Verification items for the finished model (mm, model axes). Coordinates: 2 decimals unless noted, no trailing zeros. Order: outer loops, then holes, each group sorted by start corner. A loop starts at its lowest first (then second) coordinate and runs counter-clockwise, first axis right, second up. Notation, with made-up numbers: (27.25, 48.5) - (68.25, 48.5) arc R11 ccw to (68.25, 69.5) - close; hole circle Ø7 at (2.25, -6.5). An arc over 180 degrees is marked (long way). Answer as CSV lines item,"result". Start each with the question number.
1. Material ranges on L1, parallel to Y at x = 42.5, z = 11.5; L2, parallel to Y at x = 49, z = 11; L3, parallel to X at y = 36, z = 4 (3 decimals), recorded low to high. Write a range as [from, to].
2. Section check B-B (y = 24). Record the cut outline in (x, z), and give its area (3 significant figures).
3. Section check C-C (x = 44). Record the cut outline in (y, z), and give its area (3 significant figures).
4. Go/stop test with flat-tipped pins: pin 1 (1.5 mm diameter, centred on x = 63, z = 41.5, fed in from +Y); pin 2 (10 mm diameter, centred on x = 50, z = 26.5, fed in from +Y); pin 3 (2 mm diameter, centred on x = 42, z = 33.5, fed in from +Y). Record where each tip stops, or that it passes through.
5. Section check D-D (y = 39). Record the cut outline in (x, z), and give its area (3 significant figures).
6. Section check A-A (z = 28.5). Record the cut outline in (x, y), and give its area (3 significant figures).
from build123d import *

# Parameters (mm, degrees)
F1_DEPTH = 50.8


with BuildPart() as f1:
    # F0 (on Top) → F1 (new body)
    with BuildSketch(Plane.XY):
        with BuildLine():
            Line((38.1, 50.8), (0, 50.8))
            Line((0, 50.8), (0, 0))
            Line((0, 0), (38.1, 0))
            Line((38.1, 0), (38.1, 12.7))
            ThreePointArc((38.1, 12.7), (25.4, 25.4), (38.1, 38.1))
            Line((38.1, 38.1), (38.1, 50.8))
        make_face()
        with BuildLine():
            Line((76.2, 25.4), (38.1, 50.8))
            Line((38.1, 50.8), (38.1, 38.1))
            ThreePointArc((38.1, 38.1), (47.080256, 34.380256), (50.8, 25.4))
            Line((50.8, 25.4), (76.2, 25.4))
        make_face()
        with BuildLine():
            Line((76.2, 0), (76.2, 25.4))
            Line((76.2, 25.4), (50.8, 25.4))
            ThreePointArc((50.8, 25.4), (47.080256, 16.419744), (38.1, 12.7))
            Line((38.1, 12.7), (38.1, 0))
            Line((38.1, 0), (76.2, 0))
        make_face()
    extrude(amount=F1_DEPTH)


solid = f1.part
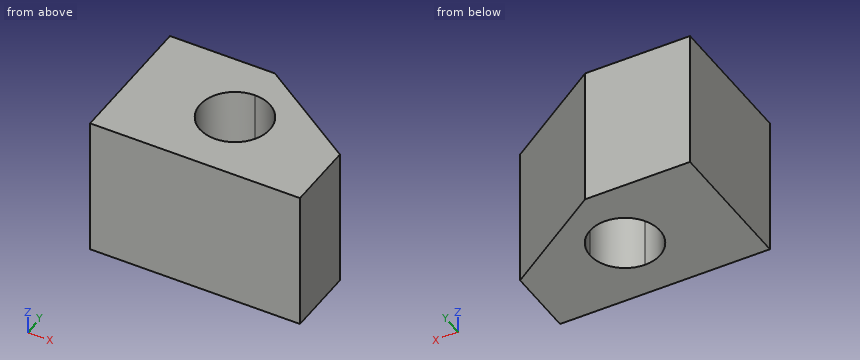
Evaluation:
1,L1,"y = [0, 13.49], [37.31, 47.87]"
1,L2,"y = [0, 18.88], [31.92, 43.53]"
1,L3,"x = [0, 31.105], [45.095, 60.3]"
2,outline,"(0, 0) - (25.48, 0) - (25.48, 50.8) - (0, 50.8) - close; (50.72, 0) - (76.2, 0) - (76.2, 50.8) - (50.72, 50.8) - close"
2,area,"2,590 mm²"
3,outline,"(0, 0) - (14.15, 0) - (14.15, 50.8) - (0, 50.8) - close; (36.65, 0) - (46.87, 0) - (46.87, 50.8) - (36.65, 50.8) - close"
3,area,"1,240 mm²"
4,pin 1,"stops at y = 34.7"
4,pin 2,"stops at y = 46.2"
4,pin 3,"stops at y = 48.87"
5,outline,"(0, 0) - (55.8, 0) - (55.8, 50.8) - (0, 50.8) - close"
5,area,"2,830 mm²"
6,outline,"(0, 0) - (76.2, 0) - (76.2, 25.4) - (38.1, 50.8) - (0, 50.8) - close; hole circle Ø25.4 at (38.1, 25.4)"
6,area,"2,880 mm²"
